Drawing for the job (mm, zero at the part's lowest x, y, z). A direction names the side the tool comes from. Coordinates: 2 decimals unless noted, no trailing zeros. Loops run counter-clockwise (first coordinate to the right, second up) from the corner with the lowest first, then second, coordinate; pieces in that order, holes last. Notation, with made-up numbers: (5.5, 62.5) - (40.5, 62.5) arc R19 ccw to (40.5, 69.5) - close; hole circle Ø5 at (49.25, 87.25). An arc over 180 degrees is marked (long way). One line per item, written item: value.
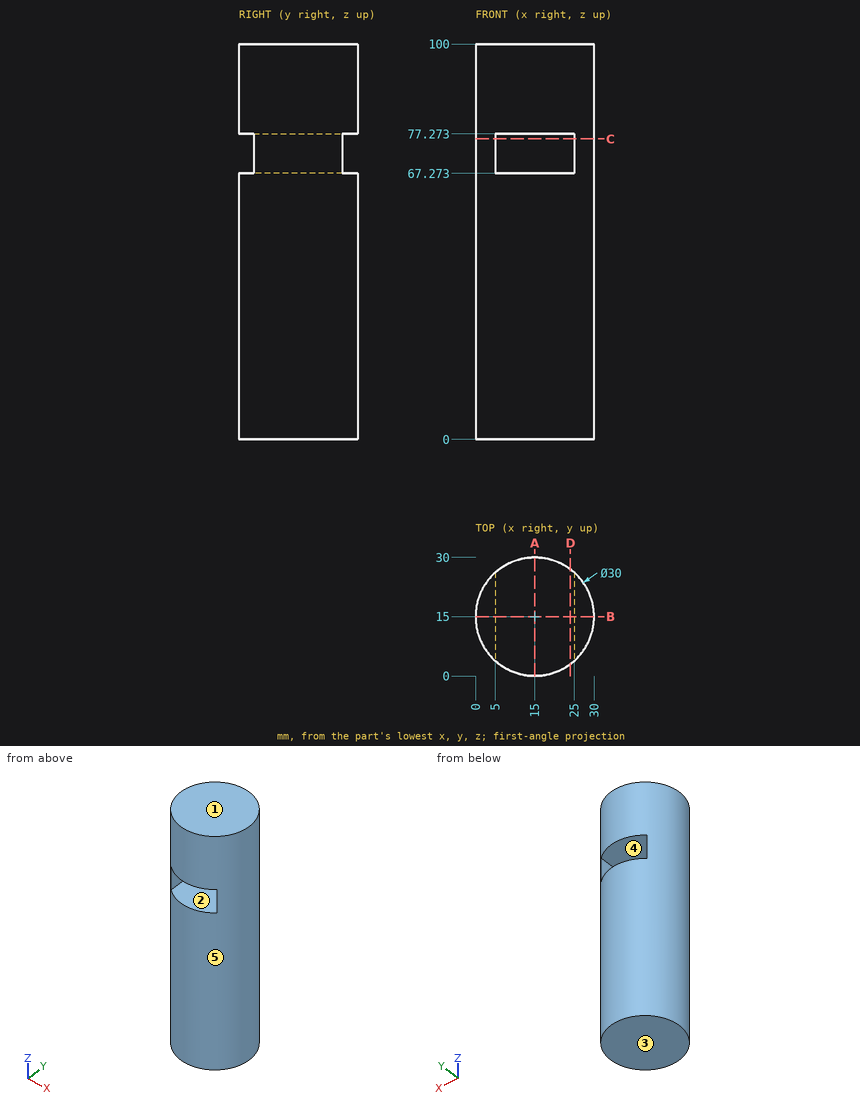
Item 1: Cut at D-D, the plane x = 24. Write the cut outline in (y, z), then the cut area to 3 significant figures.
Check result:
outline: (3, 0) - (27, 0) - (27, 67.27) - (3, 67.27) - close; (3, 77.27) - (27, 77.27) - (27, 100) - (3, 100) - close
area: 2,160 mm^2
Item 2: Tool access for the marked faces 4 and 5: list every direction of +Z, -Z, +X, -X, +Y, -Y with a clear straight run to the whole face (end or side of a thin tool).
Check result:
face 4: +Y, -Y
face 5: +Z, -Z
Item 3: Cut at A-A, the plane x = 15. Write the cut outline in (y, z).
Check result:
outline: (0, 0) - (30, 0) - (30, 67.27) - (0, 67.27) - close; (0, 77.27) - (30, 77.27) - (30, 100) - (0, 100) - close
Item 4: Cut at C-C, the plane z = 76. Write the cut outline in (x, y), then the cut area to 3 significant figures.
Check result:
outline: (5, 3.82) - (5, 26.18) arc R15 ccw to start; (25, 3.82) arc R15 ccw to (25, 26.18) - close
area: 155 mm^2
Item 5: Probe probe 1 along Z at (x, y) = (24.5, 8.75); probe 2 along X at (y, z) = (25, 31); probe 3 along X at (y, z) = (15.25, 48). List the from-to ranges inside material, lowest first. Write a range as from..to.
Check result:
probe 1: z = 0..67.27, 77.27..100
probe 2: x = 3.82..26.18
probe 3: x = 0..30
Item 6: Cut at B-B, the plane y = 15. Write the cut outline in (x, z).
Check result:
outline: (0, 0) - (30, 0) - (30, 100) - (0, 100) - close; hole (5, 67.27) - (25, 67.27) - (25, 77.27) - (5, 77.27) - close
Item 7: Drop flat-ended pins along their axis: P1, Ø5, axis at y = 18.5, z = 71.5, coming from the -X side; P2, Ø8, axis at y = 20.5, z = 54.5, coming from the +X side (1 decimal); P3, Ø3, axis at x = 9, z = 64.5, coming from the +Y side; P4, Ø4, axis at x = 16.5, z = 71, coming from the -Y side. Give the stop position or say it passes through.
Check result:
P1: stops at x = 0.03
P2: stops at x = 29.9
P3: stops at y = 29.31
P4: passes through
Item 8: Pull direction Z, two halves, no side cores. Call the marked faces 1, 2 and 3: released by +Z, released by -Z, zero draft, split by the parting line, or undercut.
Check result:
face 1: released by +Z
face 2: undercut
face 3: released by -Z
